Here's the drawing with two shaded views (mm, measured from the low corner). I have some questions. A direction names the side the tool comes from. Round coordinates to 2 decimals unless told otherwise and drop trailing zeros. Order: outer loops, then holes, each group sorted by start corner. A loop starts at its lowest first (then second) coordinate and runs counter-clockwise, first axis right, second up.
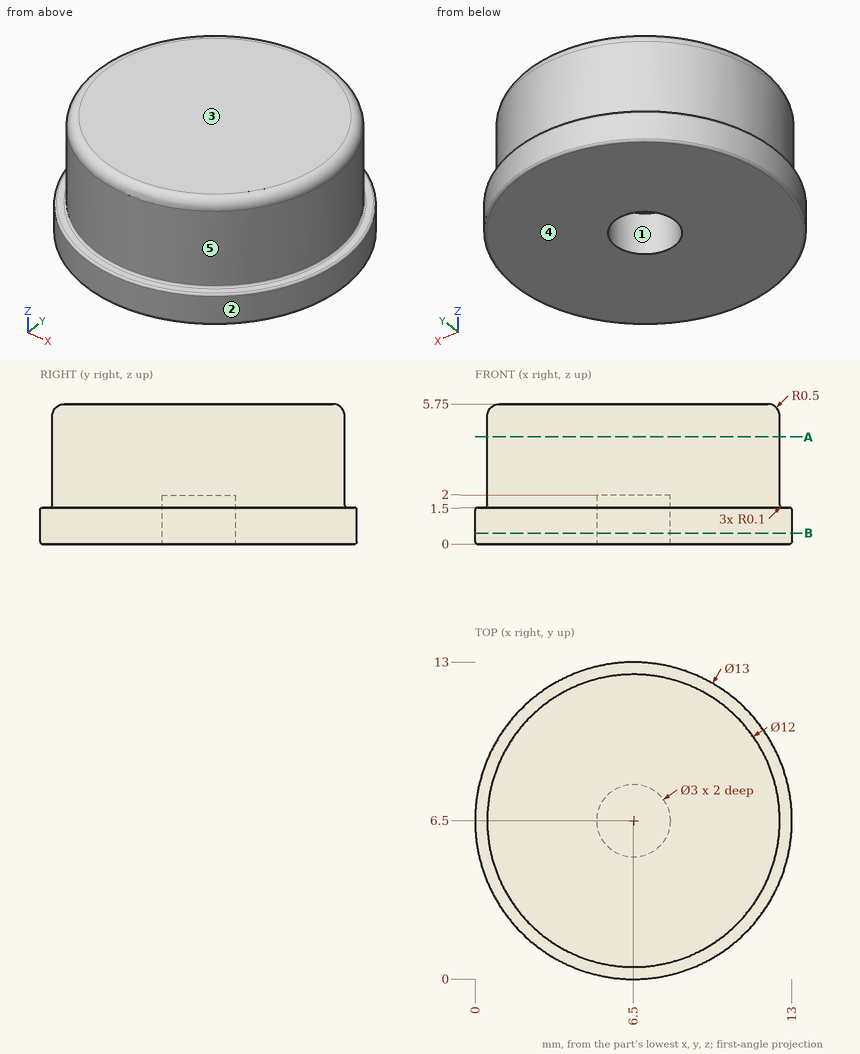
1. If we mould it in two halves opening along Y, with no side actions, what happens to the marked faces 1, 2 and 3? For each: released by +Y, released by -Y, zero draft, split by the parting line, or undercut.
Evaluation:
face 1: undercut
face 2: split by the parting line
face 3: zero draft
2. I need wall thicknesses on probe 1 along Y at (x, z) = (6.5, 1.2); probe 2 along Z at (x, y) = (6.75, 7); probe 3 along Y at (x, z) = (6, 0.6). Which ranges of each line are inside material? Lowest first, please.
Evaluation:
probe 1: y = 0 to 5, 8 to 13
probe 2: z = 2 to 5.75
probe 3: y = 0.02 to 5.09, 7.91 to 12.98
3. I'm going to push a flat-ended pin straight in: P1, Ø3, axis at x = 2, z = 3.5, coming from the -Y side. Where does the tip first touch, or does it pass through?
Evaluation:
P1: stops at y = 1.3
4. On a 3-axis mill with a long thin cutter (end or side, diameter ignored), from which of +Z, -Z, +X, -X, +Y, -Y can I reach the whole of each face in a straight line? I mean the marked faces 4 and 5. Say none if no direction works.
Evaluation:
face 4: -Z, +X, -X, +Y, -Y
face 5: +Z
5. If we section it at B-B, the plane z = 0.45: Write out the boundary of the cut face in (x, y).
Evaluation:
outline: circle Ø13 at (6.5, 6.5); hole circle Ø3 at (6.5, 6.5)
6. If we section it at A-A, the plane z = 4.4: Write out the boundary of the cut face in (x, y), and give its area (3 significant figures).
Evaluation:
outline: circle Ø12 at (6.5, 6.5)
area: 113 mm2
